Could you check a few things on this model? Use its own coordinates, in mm. Give positions to 0.01 mm unless a question says otherwise; leave off trailing zeros. Loops run counter-clockwise (first coordinate to the right, second up) from the corner with the lowest first, then second, coordinate; pieces in that order, holes last.
1. Thinking about a two-plate mould opening in Y: for faces 1 (the flat face through (286, 39, 20)), 2 (the flat face through (286, 10, 19)), 3 (the flat face through (286, 60, 14)), which applies, +Y half, -Y half, draft (parallel to the pull), parting line (faces both ways), or undercut?
2. I need wall thicknesses on line 1 along X through (y, z) = (37, 13.25); line 2 along Y through (x, z) = (422.5, 6); line 3 along Y through (x, z) = (555, 12.5). Which ranges of each line are inside material? Lowest first, please.
3. For P1, Ø5, axis at x = 25, y = 37, coming from the -Z side; P2, Ø9.5, axis at x = 290, y = 37, coming from the +Z side; P3, Ø4, axis at x = 153, z = 23, coming from the -Y side, each with a flat end and sliding along its axis, tell me the tip position at first contact or that it passes through.
4. Imagine slicing it at A-A (z = 15.5). List the corners of the cut face in (x, y) for me, plus the area to 3 significant figures.
5. Imagine slicing it at B-B (x = 275.5). List the corners of the cut face in (y, z) for me.
6. Imagine slicing it at C-C (y = 12). List the corners of the cut face in (x, z) for me, plus the area to 3 significant figures.
Autodesk Inventor part; units mm, degrees
ref_plane "YZ Plane" through (0, 0, 0) normal (1, 0, 0) x (0, 1, 0)
ref_plane "XZ Plane" through (0, 0, 0) normal (0, 1, 0) x (-1, 0, 0)
ref_plane "XY Plane" through (0, 0, 0) normal (0, 0, 1) x (1, 0, 0)
sketch "草圖1" plane through (0, 0, 0) normal (1, 0, 0) x (0, 1, 0)
  line L0 (-12, 0) -> (72, 0)
  line L1 (0, -5.6) -> (0, 33.6)
  line L2 (0, 0) -> (60, 0)
  line L3 (60, 0) -> (60, 28)
  line L4 (0, 9) -> (0, 0)
  line L5 (45, 28) -> (29, 28)
  line L6 (29, 28) -> (29, 20)
  line L7 (29, 20) -> (45, 20)
  line L8 (45, 20) -> (45, 28)
  line L9 (19, 28) -> (0, 9)
  line L10 (60, 28) -> (19, 28)
  dimension "d1" = 28
  dimension "d2" = 15
  dimension "d3" = 8
  dimension "d4" = 16
  dimension "d6" = 10
extrude "擠出1" add sketch "草圖1" along normal blind 580 contours L1 L9 L10 L6 L7 L8 L3 L0
fillet "圓角1" radius 5 1 edges at (290, 0, 0)
sketch "草圖2" plane through (0, 29, 20) normal (0, 0, 1) x (1, 0, 0)
  line L0 (-116, -29) -> (696, -29)
  line L1 (0, -41) -> (0, 43)
  line L2 (0, 31) -> (580, 31)
  line L3 (0, 8) -> (580, 8)
  point P0 (0, -29)
  point P1 (555, 8)
  point P2 (422.5, 8)
  point P3 (290, 8)
  point P4 (157.5, 8)
  point P5 (25, 8)
  point P6 (580, 0)
  dimension "d10" = 23
  dimension "d11" = 25
  dimension "d12" = 132.5
  dimension "d13" = 132.5
  dimension "d14" = 132.5
  dimension "d15" = 132.5
hole "孔1" at (555, 37, 20) at (422.5, 37, 20) at (290, 37, 20) at (157.5, 37, 20) at (25, 37, 20) at (580, 29, 20) direction (0, 0, -1) diameter 8.376 end through all
delete faces "刪除面1" heal yes whole lump no faces at (575.812, 29, 6.6667)
properties part number "exercise3-13"
Derived:
1. face 1: undercut
1. face 2: -Y half
1. face 3: +Y half
2. line 1: x = 0 to 20.81, 29.19 to 153.31, 161.69 to 285.81, 294.19 to 418.31, 426.69 to 550.81, 559.19 to 580
2. line 2: y = 0 to 32.81, 41.19 to 60
2. line 3: y = 3.5 to 32.81, 41.19 to 60
3. P1: passes through
3. P2: stops at z = 20
3. P3: stops at y = 12
4. outline: (0, 6.5) - (580, 6.5) - (580, 60) - (0, 60) - close; hole circle Ø8.38 at (25, 37); hole circle Ø8.38 at (157.5, 37); hole circle Ø8.38 at (290, 37); hole circle Ø8.38 at (422.5, 37); hole circle Ø8.38 at (555, 37)
4. area: 30,800 mm2
5. outline: (0, 5) arc R5 ccw to (5, 0) - (60, 0) - (60, 28) - (45, 28) - (45, 20) - (29, 20) - (29, 28) - (19, 28) - (0, 9) - close
6. outline: (0, 0) - (580, 0) - (580, 21) - (0, 21) - close
6. area: 12,200 mm2
